Work out the finished part from the listing and answer in its coordinate system (mm). A direction names the side the tool comes from. Give positions to 0.01 mm unless a question says otherwise; leave off trailing zeros. Loops run counter-clockwise (first coordinate to the right, second up) from the corner with the lowest first, then second, coordinate; pieces in that order, holes last. Notation, with made-up numbers: M 33,29 L 76,29 A19 cw 76,52 Z; hole C 44,53.25 d4. An arc over 180 degrees is marked long. Answer as a JSON object with one key per item and string values. Group by question number.
Autodesk Inventor part; units mm, degrees
ref_plane "YZ Plane" through (0, 0, 0) normal (1, 0, 0) x (0, 1, 0)
ref_plane "XZ Plane" through (0, 0, 0) normal (0, 1, 0) x (-1, 0, 0)
ref_plane "XY Plane" through (0, 0, 0) normal (0, 0, 1) x (1, 0, 0)
ref_plane "작업 평면1" through (0, 0, 0) normal (0, 0, 1) x (1, 0, 0)
sketch "스케치1" plane through (0, 0, 0) normal (0, 0, 1) x (1, 0, 0)
  circle A0 centre (-5.6569, -5.6569) radius 1.2
  circle A1 centre (5.6569, -5.6569) radius 1.2
  circle A2 centre (5.6569, 5.6569) radius 1.2
  circle A3 centre (-5.6569, 5.6569) radius 1.2
  circle A4 centre (0, 0) radius 4
  circle A5 centre (0, 0) radius 10.9
  circle A6 centre (0, 8) radius 1.2
  circle A7 centre (8, 0) radius 1.2
  circle A8 centre (0, -8) radius 1.2
  circle A9 centre (-8, 0) radius 1.2
  line L0 (10.9, 0) -> (10.9, 10.9)
  line L1 (10.9, 10.9) -> (-10.9, 10.9)
  line L2 (-10.9, 10.9) -> (-10.9, 0)
  line L3 (-10.9, 10.9) -> (10.9, 10.9)
  line L4 (10.9, 80.9) -> (-10.9, 80.9)
  line L5 (10.9, 80.9) -> (25.9, 80.9)
  line L6 (25.9, 80.9) -> (10.9, 10.9)
  line L7 (-10.9, 80.9) -> (-25.9, 80.9)
  line L8 (-25.9, 80.9) -> (-10.9, 10.9)
  circle A10 centre (0, 72.9) radius 1.35
  circle A11 centre (0, 48.9) radius 1.35
  line L9 (-3.05, 54.85) -> (3.05, 54.85)
  line L10 (3.05, 54.85) -> (3.05, 66.95)
  line L11 (3.05, 66.95) -> (-3.05, 66.95)
  line L12 (-3.05, 66.95) -> (-3.05, 54.85)
  line L13 (-3.05, 54.85) -> (3.05, 66.95) construction
  line L14 (3.05, 54.85) -> (-3.05, 66.95) construction
  circle A12 centre (0, 0) radius 4.1
  circle A13 centre (5.6569, 5.6569) radius 1.25
  circle A14 centre (0, 8) radius 1.25
  circle A15 centre (-5.6569, 5.6569) radius 1.25
  circle A16 centre (-8, 0) radius 1.25
  circle A17 centre (-5.6569, -5.6569) radius 1.25
  circle A18 centre (0, -8) radius 1.25
  circle A19 centre (5.6569, -5.6569) radius 1.25
  circle A20 centre (8, 0) radius 1.25
  circle A21 centre (0, 0) radius 10.9
  line L15 (-4.1, 0) -> (-4.1, -10.0995)
  line L16 (4.1, 0) -> (4.1, -10.0995)
  point P0 (0, 0)
  point P1 (0, 60.9)
  dimension "d22" = 2.7
  dimension "d23" = 2.7
  dimension "d28" = 6.1
  dimension "d29" = 12.1
  dimension "d33" = 2.5
  dimension "d36" = 360
extrude "돌출6" add sketch "스케치1" along normal blind 6 contours A5 L16 A12 L15 | L2 L1 A5 | L1 L0 A5 | L1 L8 L7 L4 L5 L6 picked at (-5.5569, -1.7483)
fillet "모깎기2" radius 1 2 edges at (4.1, -10.0995, 3) (-4.1, -10.0995, 3)
fillet "모깎기3" radius 2 2 edges at (25.9, 80.9, 3) (-25.9, 80.9, 3)
sketch "스케치2" plane through (0, 0, 6) normal (0, 0, 1) x (1, 0, 0)
  line L0 (3.05, 66.95) -> (3.05, 54.85)
  line L1 (-3.05, 54.85) -> (-3.05, 66.95)
  line L2 (-3.05, 66.95) -> (3.05, 66.95)
  line L3 (3.05, 54.85) -> (-3.05, 54.85)
  circle A0 centre (3.05, 66.95) radius 1
  circle A1 centre (-3.05, 66.95) radius 1
  circle A2 centre (-3.05, 54.85) radius 1
  circle A3 centre (3.05, 54.85) radius 1
  point P0 (0, 0)
  dimension "d42" = 2
  dimension "d43" = 2
  dimension "d44" = 2
  dimension "d45" = 2
extrude "돌출7" cut sketch "스케치2" against normal blind 10 contours L2 A0 L0 | L0 A0 L2 | A3 L3 L0 | L0 L3 A3 | A1 L1 L2 | L2 L1 A1 | A2 L1 L3 | L3 L1 A2
properties part number "hand" material "PMMA 플라스틱"
Item 1: A cutting plane is placed at B-B (x = 0). Determine the outline of the cut face in (y, z).
Item 2: A cutting plane is placed at A-A (y = 8). Determine the outline of the cut face in (x, z).
Item 3: A tool of negligible diameter and unlimited length cuts with its end or side. For faces 1 (the flat face through (4.1, -4, 3)), 2 (the cylindrical face through (-9.448, -5.435, 2.958)), 3 (the flat face through (0, 54.85, 3)), 4 (the flat face through (10.9, 5, 3)), from which of +Z, -Z, +X, -X, +Y, -Y can it reach the whole face along a straight path? Write none if from no direction.
Item 4: Given pin 1 Ø2 at (x, y) = (0, 48.9) entering from +Z; pin 2 Ø1 at (y, z) = (59, 3) entering from +X; pin 3 Ø2 at (y, z) = (12.5, 2) entering from -X; pin 4 Ø2 at (y, z) = (19.5, 3.5) entering from +X, each flat-ended and moving along its own axis, determine where each tip first touches the part or whether it passes through.
Item 5: A cutting plane is placed at D-D (x = -8). Determine the outline of the cut face in (y, z), and give its area (3 significant figures).
Item 6: A cutting plane is placed at C-C (z = 3.45). Give the number of separate pieces and of enclosed holes in the cut face, and give its area (3 significant figures).
Item 7: Find the intervals of material crossed by probe 1 along Y at (x, z) = (0, 4.7); probe 2 along Y at (x, z) = (-1, 4.6); probe 3 along X at (y, z) = (72.9, 3.2), in increasing order. Write a range as [from, to].
Item 8: For a pull along X with two mould halves and no side action, classify faces 5 (the cylindrical face through (24.997, 80.138, 3.042)), 6 (the flat face through (0, 46, 6)), 7 (the cylindrical face through (3.78, 67.633, 3.042)), 8 (the cylindrical face through (-24.966, 80.177, 3.042)) as pulls with the +X half, pulls with the -X half, needs draft (parallel to the pull), parting line crosses it, or undercut.
The answers:
{
 "1": {"outline": "M 4.1,0 L 6.75,0 L 6.75,6 L 4.1,6 Z; M 9.25,0 L 47.55,0 L 47.55,6 L 9.25,6 Z; M 50.25,0 L 54.85,0 L 54.85,6 L 50.25,6 Z; M 66.95,0 L 71.55,0 L 71.55,6 L 66.95,6 Z; M 74.25,0 L 80.9,0 L 80.9,6 L 74.25,6 Z"},
 "2": {"outline": "M -10.9,0 L -1.25,0 L -1.25,6 L -10.9,6 Z; M 1.25,0 L 10.9,0 L 10.9,6 L 1.25,6 Z"},
 "3": {"face 1": "+Z, -Z, -Y", "face 2": "+Z, -Z, -X, -Y", "face 3": "+Z, -Z", "face 4": "+Z, -Z, +X, -Y"},
 "4": {"pin 1": "passes through", "pin 2": "stops at x = 21.31", "pin 3": "stops at x = -11.46", "pin 4": "stops at x = 12.96"},
 "5": {"outline": "M -7.4,0 L -1.25,0 L -1.25,6 L -7.4,6 Z; M 1.25,0 L 80.9,0 L 80.9,6 L 1.25,6 Z", "area": "515 mm^2"},
 "6": {"separate pieces": "1", "enclosed holes": "10", "area": "2,750 mm^2"},
 "7": {"probe 1": "y = [4.1, 6.75], [9.25, 47.55], [50.25, 54.85], [66.95, 71.55], [74.25, 80.9]", "probe 2": "y = [3.98, 7.25], [8.75, 47.99], [49.81, 54.85], [66.95, 71.99], [73.81, 80.9]", "probe 3": "x = [-24.19, -1.35], [1.35, 24.19]"},
 "8": {"face 5": "pulls with the +X half", "face 6": "needs draft", "face 7": "undercut", "face 8": "pulls with the -X half"}
}
